```python
from build123d import *

# Parameters (mm, degrees)
SKETCH1_R                                      = 0.5
SKETCH1_R_2                                    = 5
BOSS_EXTRUDE1_DEPTH                            = 5
BOSS_EXTRUDE4_DEPTH                            = 5.7
BOSS_EXTRUDE4_DEPTH_BACK                       = 0.5
SKETCH3_R                                      = 1.3
BOSS_EXTRUDE6_DEPTH                            = 1
FILLET1_R                                      = 2.5
FILLET2_R                                      = 2
F_2_0MM_DOWEL_HOLE1_D                          = 2
F_2_0MM_DOWEL_HOLE1_DEPTH                      = 42.93
F_2_0MM_DOWEL_HOLE1_TIP                        = 0.600860619
SKETCH12_R                                     = 2.75
SKETCH12_R_2                                   = 2.625
CUT_EXTRUDE1_DEPTH                             = 10
CSK_FOR_M2_5_FLAT_HEAD_MACHINE_SCREW1_AT_COUNT = 2
CSK_FOR_M2_5_FLAT_HEAD_MACHINE_SCREW1_AT_PITCH = 28


with BuildPart() as part:
    # Sketch1 → Boss-Extrude1 (new body)
    with BuildSketch(Plane(origin=(0, 0, 0), x_dir=(1, 0, 0), z_dir=(0, 1, 0))):
        with BuildLine():
            Line((1.767766953, 14.596194078), (14.596194078, 1.767766953))
            ThreePointArc((14.596194078, 1.767766953), (15.328427125, 0), (14.596194078, -1.767766953))
            Line((14.596194078, -1.767766953), (1.767766953, -14.596194078))
            ThreePointArc((1.767766953, -14.596194078), (0, -15.328427125), (-1.767766953, -14.596194078))
            Line((-1.767766953, -14.596194078), (-14.596194078, -1.767766953))
            ThreePointArc((-14.596194078, -1.767766953), (-15.328427125, 0), (-14.596194078, 1.767766953))
            Line((-14.596194078, 1.767766953), (-1.767766953, 14.596194078))
            ThreePointArc((-1.767766953, 14.596194078), (0, 15.328427125), (1.767766953, 14.596194078))
        make_face()
        with Locations(Location((0, 10, 0), (0, 0, 270))):
            Circle(SKETCH1_R, mode=Mode.SUBTRACT)
        with Locations(Location((0, -10, 0), (0, 0, 270))):
            Circle(SKETCH1_R, mode=Mode.SUBTRACT)
        with Locations(Location((10, 0, 0), (0, 0, 270))):
            Circle(SKETCH1_R, mode=Mode.SUBTRACT)
        with Locations(Location((-10, 0, 0), (0, 0, 270))):
            Circle(SKETCH1_R, mode=Mode.SUBTRACT)
        with Locations(Location((0, 0, 0), (0, 0, 270))):
            Circle(SKETCH1_R_2, mode=Mode.SUBTRACT)
    extrude(amount=BOSS_EXTRUDE1_DEPTH)

    # Sketch3 → Boss-Extrude4 (add, two sides: drawn at the far end of the back side and taken through both)
    # profile 1 of 4: a face of its own
    with BuildSketch(Plane(origin=(0, -2.7, 0), x_dir=(1, 0, 0), z_dir=(0, 1, 0)).offset(-BOSS_EXTRUDE4_DEPTH_BACK)):
        Polygon((-4.949747468, -10.537489101), (-0.637994164, -14.849242405), (-4.949747468, -19.160995709), (-9.261500772, -14.849242405), align=None)
        with Locations(Location((-4.949747468, -14.849242405, 0), (0, 0, 270))):
            Circle(SKETCH3_R, mode=Mode.SUBTRACT)
    # profile 2 of 4: a face of its own
    with BuildSketch(Plane(origin=(0, -2.7, 0), x_dir=(1, 0, 0), z_dir=(0, 1, 0)).offset(-BOSS_EXTRUDE4_DEPTH_BACK)):
        Polygon((-6.717514421, -8.769722148), (-11.029267725, -13.081475452), (-9.261500772, -14.849242405), (-4.949747468, -10.537489101), align=None)
    # profile 3 of 4: a face of its own
    with BuildSketch(Plane(origin=(0, -2.7, 0), x_dir=(1, 0, 0), z_dir=(0, 1, 0)).offset(-BOSS_EXTRUDE4_DEPTH_BACK)):
        Polygon((19.160995709, 4.949747468), (14.849242405, 9.261500772), (10.537489101, 4.949747468), (14.849242405, 0.637994164), align=None)
        with Locations(Location((14.849242405, 4.949747468, 0), (0, 0, 270))):
            Circle(SKETCH3_R, mode=Mode.SUBTRACT)
    # profile 4 of 4: a face of its own
    with BuildSketch(Plane(origin=(0, -2.7, 0), x_dir=(1, 0, 0), z_dir=(0, 1, 0)).offset(-BOSS_EXTRUDE4_DEPTH_BACK)):
        Polygon((13.081475452, 11.029267725), (14.849242405, 9.261500772), (10.537489101, 4.949747468), (8.769722148, 6.717514421), align=None)
    extrude(amount=BOSS_EXTRUDE4_DEPTH + BOSS_EXTRUDE4_DEPTH_BACK)


with BuildPart() as boss_extrude6_tool:
    # Sketch7 → Boss-Extrude6 (new body)
    with BuildSketch(Plane(origin=(2.525126055, -2.13e-07, 2.525126055), x_dir=(0.7071067811865474, 0, -0.7071067811865477), z_dir=(0.7071067811865465, -5.960464483662305e-08, 0.7071067811865461))):
        Polygon((11.571067812, 5.000000541), (17.04887, 3.00000056), (11.571067812, 3.000000541), align=None)
        Polygon((-11.571067812, 5.000000541), (-17.04887, 3.00000056), (-11.571067812, 3.000000541), align=None)
    extrude(amount=-BOSS_EXTRUDE6_DEPTH)


with BuildPart() as part_1:
    add(part.part)


with BuildPart() as part_2:
    # Boss-Extrude6: joined with boss_extrude6_tool
    add(part_1.part.fuse(boss_extrude6_tool.part, tol=0.00001))

    # Fillet1
    fillet1_edges = [part_2.edges().sort_by_distance(p)[0] for p in [
        (-7.155876652, 1.5, 9.208084379),
        (-0.935534875, 1.5, 15.146783115),
        (9.208084379, 1.5, -7.155876652),
        (15.146783115, 1.5, -0.935534875),
    ]]
    fillet(fillet1_edges, radius=FILLET1_R)

    # Fillet2
    # the kernel refuses this fillet: 2 mm, written as the material it takes off along each edge
    with BuildSketch(Plane(origin=(-4.949747468, 8, 19.160995709), x_dir=(0.7071067811865477, 0, -0.7071067811865475), z_dir=(0, -1, 0)), Plane(origin=(-11.029267725, -8.2, 13.081475452), x_dir=(0.7071067811865476, 0, -0.7071067811865476), z_dir=(0, 1, 0))) as fillet2_piece_1:
        with BuildLine():
            CenterArc((FILLET2_R, -FILLET2_R), FILLET2_R, 90, 90)
            Line((0, -FILLET2_R), (0, 0))
            Line((0, 0), (FILLET2_R, 0))
        make_face()
    extrude(amount=16.2, mode=Mode.SUBTRACT)
    with BuildSketch(Plane(origin=(13.081475452, -8.2, -11.029267725), x_dir=(-0.7071067811865471, 0, 0.707106781186548), z_dir=(0, 1, 0)), Plane(origin=(19.160995709, 8, -4.949747468), x_dir=(-0.7071067811865472, 0, 0.7071067811865477), z_dir=(0, -1, 0))) as fillet2_piece_2:
        with BuildLine():
            CenterArc((FILLET2_R, FILLET2_R), FILLET2_R, 180, 90)
            Line((0, FILLET2_R), (0, 0))
            Line((0, 0), (FILLET2_R, 0))
        make_face()
    extrude(amount=16.2, mode=Mode.SUBTRACT)

    # Ø2.0mm Dowel Hole1
    with Locations(Plane.XZ):
        with Locations((0, 10), (10, 0), (-10, 0), (0, -10)):
            Hole(F_2_0MM_DOWEL_HOLE1_D / 2, depth=F_2_0MM_DOWEL_HOLE1_DEPTH)
            with Locations((0, 0, -(F_2_0MM_DOWEL_HOLE1_DEPTH + F_2_0MM_DOWEL_HOLE1_TIP / 2))):  # 118° drill point
                Cone(0, F_2_0MM_DOWEL_HOLE1_D / 2, F_2_0MM_DOWEL_HOLE1_TIP, mode=Mode.SUBTRACT)

    # Sketch12 → Cut-Extrude1 (cut)
    with BuildSketch(Plane(origin=(0, 3, 0), x_dir=(1, 0, 0), z_dir=(0, 1, 0))):
        with Locations((-4.949747468, -14.849242405)):
            Circle(SKETCH12_R)
        with Locations((14.849242405, 4.949747468)):
            Circle(SKETCH12_R_2)
    extrude(amount=CUT_EXTRUDE1_DEPTH, mode=Mode.SUBTRACT)

    # Sketch13 → CSK for M2.5 Flat Head Machine Screw1 (revolve, cut)
    with BuildSketch(Plane(origin=(-4.949747468, 3, 14.849242405), x_dir=(0, 0, 1), z_dir=(1, 0, 0))):
        Polygon((0, 0), (0, 43.741161836), (1.35, 42.93), (1.35, 1.4), (2.75, 0), align=None)
    csk_for_m2_5_flat_head_machine_screw1 = revolve(axis=Axis((-4.949747468, 9.35, 14.849242405), (0, -1, 0)), mode=Mode.SUBTRACT)

    # CSK for M2.5 Flat Head Machine Screw1 at: CSK for M2.5 Flat Head Machine Screw1 ×2
    with Locations(*[Vector(0.7071067811865477, 0, -0.7071067811865475) * (i * CSK_FOR_M2_5_FLAT_HEAD_MACHINE_SCREW1_AT_PITCH) for i in range(1, CSK_FOR_M2_5_FLAT_HEAD_MACHINE_SCREW1_AT_COUNT)]):
        add(csk_for_m2_5_flat_head_machine_screw1, mode=Mode.SUBTRACT)


solid = part_2.part
```
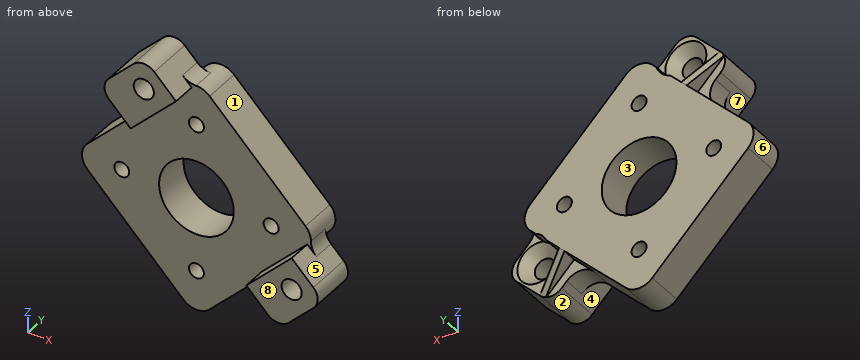
Model file for the job. Use its own axes, mm. Face numbers are marked on the shaded views. A direction names the side the tool comes from. Round coordinates to 2 decimals unless told otherwise and drop trailing zeros. Write each loop counter-clockwise with the first axis right and the second up, starting at its lowest first coordinate (ties: lowest second). Pieces come first, ordered by that corner, then holes. Notation, with made-up numbers: (12.25, -39) -> (64.25, -39) arc R17 cw to (64.25, -8) -> close; hole circle Ø2 at (27.5, -30). An arc over 180 degrees is marked (long way). Answer as CSV lines item,"result".
1. Pin check, flat tips, straight feed: pin 1 Ø3 at (x, z) = (-4.95, 14.85) entering from +Y; pin 2 Ø9.5 at (x, z) = (3, 7.5) entering from -Y; pin 3 Ø3 at (y, z) = (-1, 1) entering from +X; pin 4 Ø6 at (x, z) = (3.5, 3.5) entering from +Y. Stop position of each tip, or through.
Resolved:
pin 1,"y = 1.75"
pin 2,"y = 0"
pin 3,"x = 15.33"
pin 4,"y = 5"
2. Slice it at C-C, the plane y = 4. List the corners of the cut face in (x, z) (3 decimals), plus the area to 3 significant figures.
Resolved:
outline,"(-14.596, -1.768) -> (-1.768, -14.596) arc R2.5 ccw to (1.768, -14.596) -> (10, -6.364) -> (11.937, -8.301) -> (12.644, -7.594) -> (10.707, -5.657) -> (12.428, -3.936) arc R2.625 cw to (13.836, -2.528) -> (14.596, -1.768) arc R2.5 ccw to (14.596, 1.768) -> (1.768, 14.596) arc R2.5 ccw to (-1.768, 14.596) -> (-2.32, 14.044) arc R2.75 cw to (-4.144, 12.22) -> (-5.657, 10.707) -> (-7.594, 12.644) -> (-8.301, 11.937) -> (-6.364, 10) -> (-14.596, 1.768) arc R2.5 ccw to start; hole circle Ø2 at (-10, 0); hole circle Ø10 at (0, 0); hole circle Ø2 at (0, -10); hole circle Ø2 at (0, 10); hole circle Ø2 at (10, 0)"
area,"444 mm²"
3. Mould opens along Z. For the marked faces 1, 2 and 3 say: +Z half, -Z half, draft (parallel to the pull), parting line (faces both ways), or undercut.
Resolved:
face 1,"+Z half"
face 2,"-Z half"
face 3,"undercut"
4. Slice it at D-D, the plane x = 7. List the corners of the cut face in (y, z).
Resolved:
outline,"(0, -9.36) -> (5, -9.36) -> (5, 9.36) -> (0, 9.36) -> close"
5. Tool access for the marked faces 4, 5, 6, 7 and 8: list every direction of +Z, -Z, +X, -X, +Y, -Y with a clear straight run to the whole face (end or side of a thin tool).
Resolved:
face 4,"-Z, -Y"
face 5,"+Z, +X, -Y"
face 6,"-X, +Y, -Y"
face 7,"-X, -Y"
face 8,"+Z, -Z, +X, -X, -Y"
6. Slice it at A-A, the plane y = -1. List the corners of the cut face in (x, z), plus the area to 3 significant figures.
Resolved:
outline,"(-9.62, 11.67) -> (-6.72, 8.77) -> (-0.64, 14.85) -> (-3.54, 17.75) arc R2 ccw to (-6.36, 17.75) -> (-9.62, 14.5) arc R2 ccw to start; (8.77, -6.72) -> (11.67, -9.62) arc R2 ccw to (14.5, -9.62) -> (17.75, -6.36) arc R2 ccw to (17.75, -3.54) -> (14.85, -0.64) -> close; hole circle Ø2.7 at (-4.95, 14.85); hole circle Ø2.7 at (14.85, -4.95)"
area,"90.0 mm²"
7. Drill centre lines: line 1 (Y direction, x = 6, z = -9); line 2 (X direction, y = 0.75, z = -2.5); line 3 (X direction, y = 2.25, z = 3). Where is each one in solid material? Low to high.
Resolved:
line 1,"0 to 5"
line 2,"-13.86 to -4.33, 4.33 to 16.71"
line 3,"-13.36 to -4, 4 to 13.36"
8. Slice it at B-B, the plane z = 2.5. List the corners of the cut face in (x, y), plus the area to 3 significant figures.
Resolved:
outline,"(-13.86, 0) -> (-4.33, 0) -> (-4.33, 5) -> (-13.86, 5) -> close; (4.33, 0) -> (13.86, 0) -> (13.86, 5) -> (4.33, 5) -> close"
area,"95.3 mm²"
